Drawing for the job (mm, zero at the part's lowest x, y, z). A direction names the side the tool comes from. Round coordinates to 2 decimals unless told otherwise and drop trailing zeros. Order: outer loops, then holes, each group sorted by start corner. A loop starts at its lowest first (then second) coordinate and runs counter-clockwise, first axis right, second up. Notation, with made-up numbers: (39.25, 34) -> (88.25, 34) arc R17 ccw to (88.25, 47) -> close; hole circle Ø7 at (-2, 77.5). An arc over 180 degrees is marked (long way). Use CSV: the item, a comma, the result in double quotes.
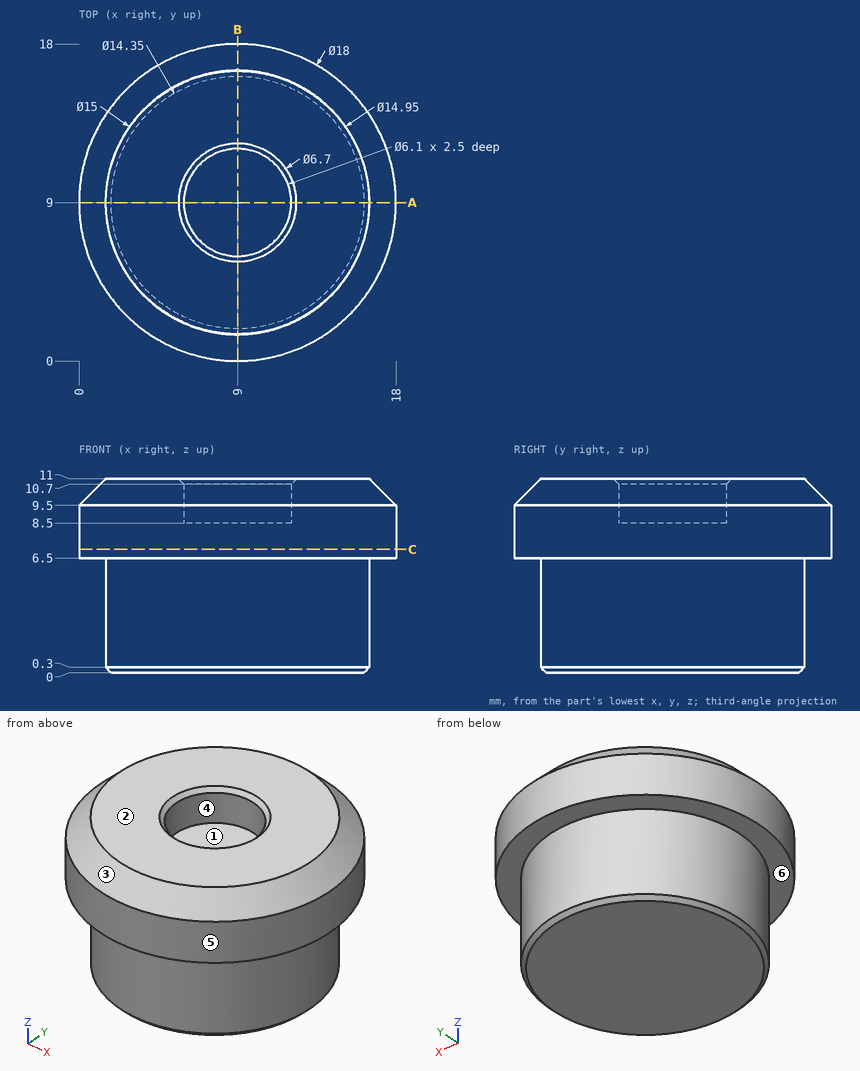
Q1. Cut at A-A (y = 9). Give the cut face in (x, z) (3 decimals).
From the geometry:
outline,"(0, 6.5) -> (1.525, 6.5) -> (1.525, 0.3) -> (1.825, 0) -> (16.175, 0) -> (16.475, 0.3) -> (16.475, 6.5) -> (18, 6.5) -> (18, 9.5) -> (16.5, 11) -> (12.35, 11) -> (12.05, 10.7) -> (12.05, 8.5) -> (5.95, 8.5) -> (5.95, 10.7) -> (5.65, 11) -> (1.5, 11) -> (0, 9.5) -> close"
Q2. Which spindle directions (+Z, -Z, +X, -X, +Y, -Y) get a long thin tool onto all of the face, cutting with end or side? Do the marked faces 5 and 6. Say none if no direction does.
From the geometry:
face 5,"+Z, -Z"
face 6,"-Z"
Q3. Pin check, flat tips, straight feed: pin 1 (6 mm diameter, centred on y = 11.5, z = 1.5, fed in from -X) (3 decimals); pin 2 (4 mm diameter, centred on y = 5, z = 3, fed in from +X); pin 3 (1 mm diameter, centred on y = 7.5, z = 9, fed in from -X). Stop position of each tip, or through.
From the geometry:
pin 1,"stops at x = 1.525"
pin 2,"stops at x = 16.2"
pin 3,"stops at x = 0.06"
Q4. Cut at C-C (z = 7). Give the cut face in (x, y).
From the geometry:
outline,"circle Ø18 at (9, 9)"
Q5. Probe line 1 along Y through (x, z) = (9, 3) (3 decimals); line 2 along Y through (x, z) = (9, 10.2); line 3 along Z through (x, y) = (7, 8). List the from-to ranges inside material, lowest first.
From the geometry:
line 1,"y = 1.525 to 16.475"
line 2,"y = 0.7 to 5.95, 12.05 to 17.3"
line 3,"z = 0 to 8.5"
Q6. Mould opens along X. For the marked faces 1, 2, 3 and 4 say: +X half, -X half, draft (parallel to the pull), parting line (faces both ways), or undercut.
From the geometry:
face 1,"undercut"
face 2,"draft"
face 3,"parting line"
face 4,"undercut"
